Read the model definition and answer for the solid it produces. Units are mm, in the model's axes. A direction names the side the tool comes from. Coordinates: 2 decimals unless noted, no trailing zeros. Order: outer loops, then holes, each group sorted by start corner. A loop starts at its lowest first (then second) coordinate and runs counter-clockwise, first axis right, second up. Notation, with made-up numbers: M 1.5,69.5 L 25.5,69.5 A26 cw 25.5,94.5 Z; hole C 26,3 d2. An arc over 180 degrees is marked long. Put each result on its own line as item: value.
Autodesk Inventor part; units mm, degrees
ref_plane "YZ Plane" through (0, 0, 0) normal (1, 0, 0) x (0, 1, 0)
ref_plane "XZ Plane" through (0, 0, 0) normal (0, 1, 0) x (-1, 0, 0)
ref_plane "XY Plane" through (0, 0, 0) normal (0, 0, 1) x (1, 0, 0)
sketch "Sketch1" plane through (0, 0, 0) normal (0, 0, 1) x (1, 0, 0)
  circle A0 centre (0, 0) radius 7.4
  dimension "d0" = 14.8
extrude "Extrusion1" add sketch "Sketch1" along normal blind 40
sketch "Sketch2" plane through (0, 0, 40) normal (0, 0, 1) x (1, 0, 0)
  line L0 (0, 0) -> (-4.9, 0)
  line L1 (0, 0) -> (4.9, 0)
  line L2 (0, 0) -> (0, 5.5)
  line L3 (0, 5.5) -> (-4.9, 5.5)
  line L4 (-4.9, 5.5) -> (-4.9, 0)
  line L5 (0, 5.5) -> (4.9, 5.5)
  line L6 (4.9, 5.5) -> (4.9, 0)
  line L7 (-4.9, 0) -> (-4.9, -10)
  line L8 (-4.9, -10) -> (4.9, -10)
  line L9 (4.9, -10) -> (4.9, 0)
  dimension "d3" = 4.9
  dimension "d4" = 4.9
  dimension "d5" = 5.5
  dimension "d6" = 10
extrude "Extrusion2" cut sketch "Sketch2" against normal blind 7.9
sketch "Sketch3" plane through (0, 0, 32.1) normal (0, 0, 1) x (1, 0, 0)
  line L0 (-4.9, -5.5453) -> (-4.9, 5.5)
  line L1 (-4.9, 5.5) -> (-4.9, 0.2)
  line L2 (-4.9, 0.2) -> (-4.1, 0.2)
  line L3 (-4.1, 0.2) -> (-4.1, -7.8)
  line L4 (-4.1, -7.8) -> (-4.9, -7.8)
  line L5 (-4.9, -7.8) -> (-4.9, 0.2)
  line L6 (4.9, 5.5) -> (4.9, -5.5453)
  line L7 (4.9, 5.5) -> (4.9, 0.2)
  line L8 (4.9, 0.2) -> (4.1, 0.2)
  line L9 (4.1, 0.2) -> (4.1, -7.8)
  line L10 (4.1, -7.8) -> (4.9, -7.8)
  line L11 (4.9, 0.2) -> (4.9, -7.8)
  point P0 (0, 0)
  dimension "d9" = 5.3
  dimension "d10" = 0.8
  dimension "d11" = 8
  dimension "d12" = 0.8
  dimension "d13" = 5.3
  dimension "d14" = 0.8
  dimension "d15" = 8
extrude "Extrusion3" cut sketch "Sketch3" against normal blind 5
sketch "Sketch4" plane through (-4.9, 5.5, 40) normal (0, -1, 0) x (1, 0, 0)
  line L0 (12.3, 0) -> (-2.5, 0)
  line L1 (6.9, 0) -> (2.9, 0)
  line L2 (4.9, 0) -> (4.9, -1.2)
  line L3 (4.9, -1.2) -> (6.9, -1.2)
  line L4 (6.9, -1.2) -> (6.9, 0)
  line L5 (4.9, -1.2) -> (2.9, -1.2)
  line L6 (2.9, -1.2) -> (2.9, 0)
  point P0 (4.9, -40)
  point P1 (9.8, 0)
  point P2 (0, 0)
  dimension "d18" = 1.2
  dimension "d19" = 2
  dimension "d20" = 2
extrude "Extrusion4" add sketch "Sketch4" along normal blind 2
sketch "Sketch5" plane through (0, 0, 0) normal (0, 1, 0) x (-1, 0, 0)
  line L0 (-7.4, 0) -> (-7.4, 40)
  line L1 (-7.4, 40) -> (-7.4, 0)
  line L2 (-7.4, 20) -> (7.4, 20)
  line L3 (7.4, 0) -> (7.4, 40)
  circle A0 centre (0, 20) radius 4
  point P0 (0, 0)
  dimension "d23" = 8
extrude "Extrusion5" add sketch "Sketch5" against normal blind 120
ref_plane "Work Plane1" through (4.9, -5.5453, 27.1) normal (0, -1, 0) x (1, 0, 0)
sketch "Sketch7" plane through (0, 0, 0) normal (0, 0, -1) x (-1, 0, 0)
  circle A0 centre (0, 0) radius 3
  dimension "d26" = 6
ref_plane "Work Plane2" through (0, 0, 0) normal (-1, 0, 0) x (0, 0, -1)
sketch "Sketch8" plane through (0, 0, 0) normal (-1, 0, 0) x (0, 0, -1)
  line L0 (0, -7.4) -> (0, 7.4)
  circle A0 centre (0, 7.4) radius 7.4
  point P0 (0, 0)
sweep "Sweep1" cut profiles "Sketch7" path "Sketch8" path curves A0
equation "\"BendRadius\" = Thickness"
equation "\"BendReliefWidth\" = Thickness"
equation "\"BendReliefDepth\" = 0.5 * Thickness"
equation "\"CornerReliefSize\" = 4 * Thickness"
equation "\"MinimumRemnant\" = 2 * Thickness"
equation "\"TransitionRadius\" = BendRadius"
equation "\"JacobiRadiusSize\" = BendRadius"
equation "\"GapSize\" = Thickness"
properties part number "rotor1"
Q1. A tool of negligible diameter and unlimited length cuts with its end or side. For faces 4 (the face through (-0.1, -3.2, 0)), 5 (the face through (-4.9, 0, 35)), from which of +Z, -Z, +X, -X, +Y, -Y can it reach the whole face along a straight path? Write none if from no direction.
Answers below:
face 4: -Z, +X, -X, +Y, -Y
face 5: +Z, -Y
Q2. Find section D-D on z = 20. Write down the section's boundary in (x, y).
Answers below:
outline: M -4,-120 L 4,-120 L 4,-6.23 A7.4 ccw long -4,-6.23 Z
Q3. Consider line 1 along Y through (x, z) = (-0.5, 34); line 2 along X through (y, z) = (-0.5, 26); line 3 along X through (y, z) = (-110, 20). Determine where each line is inside the solid, lowest interval first.
Answers below:
line 1: y = 5.5 to 7.38
line 2: x = -7.38 to 7.38
line 3: x = -4 to 4
Q4. Given pin 1 (0.6 mm diameter, centred on y = 4.5, z = 39.5, fed in from -X); pin 2 (4 mm diameter, centred on x = -4, y = -35.5, fed in from +Z); pin 3 (3.5 mm diameter, centred on y = 2, z = 34.5, fed in from -X); pin 4 (0.9 mm diameter, centred on x = -4.5, y = -2.5, fed in from +Z), each flat-ended and moving along its own axis, determine where each tip first touches the part or whether it passes through.
Answers below:
pin 1: stops at x = -6.09
pin 2: stops at z = 23.46
pin 3: stops at x = -7.4
pin 4: stops at z = 40
Q5. Find section C-C on y = -63.5. Write down the section's boundary in (x, z).
Answers below:
outline: C 0,20 d8
Q6. Find section B-B on z = 12.5. Write down the section's boundary in (x, y).
Answers below:
outline: C 0,0 d14.8
Q7. Find section A-A on x = 0. Write down the section's boundary in (y, z).
Answers below:
outline: M -120,16 L -7.4,16 L -7.4,10.4 A10.4 cw 3,0 L 7.4,0 L 7.4,40 L 3.5,40 L 3.5,38.8 L 5.5,38.8 L 5.5,32.1 L -7.4,32.1 L -7.4,24 L -120,24 Z; M -7.4,0 L -3,0 A4.4 ccw -7.4,4.4 Z
Q8. For a pull along X with two mould halves and no side action, classify faces 1 (the face through (0, -120, 20)), 2 (the face through (-4.1, -3, 30)), 3 (the face through (0.521, -62.316, 23.966)) as +X half, -X half, draft (parallel to the pull), parting line (faces both ways), or undercut.
Answers below:
face 1: draft
face 2: undercut
face 3: parting line
